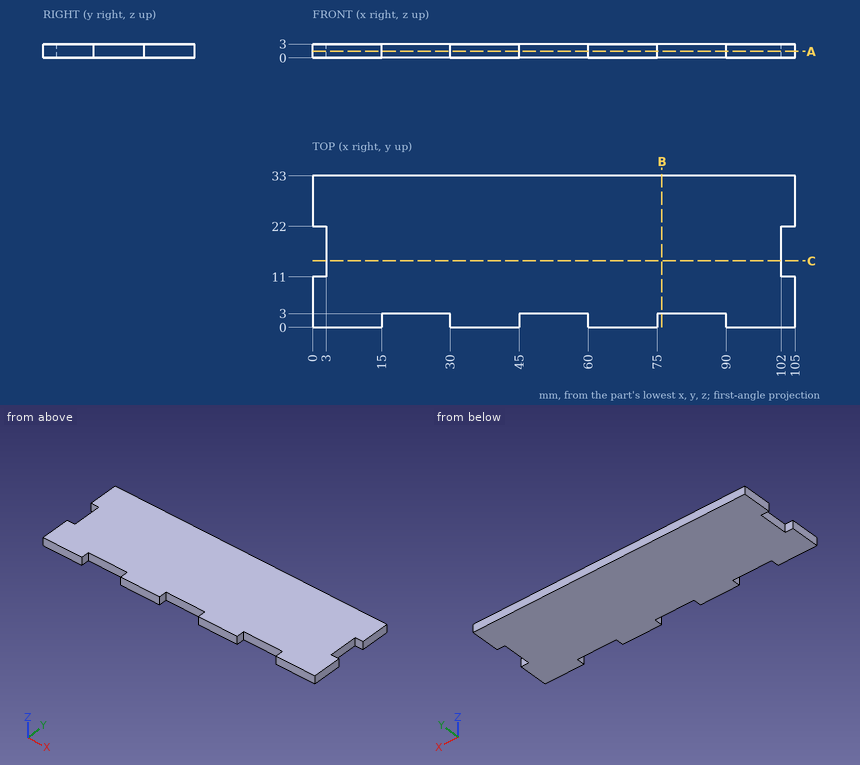
Verification items for this drawing (mm, ordinates from the low corner). Round coordinates to 2 decimals unless told otherwise and drop trailing zeros. Loops run counter-clockwise (first coordinate to the right, second up) from the corner with the lowest first, then second, coordinate; pieces in that order, holes last. Notation, with made-up numbers: (67.25, -5) - (87.25, -5) arc R17 cw to (87.25, 28) - close; hole circle Ø6 at (77, -6.75). An arc over 180 degrees is marked (long way). Answer as CSV lines item,"result". Start each with the question number.
Item 1: Scan lines: line 1 (X direction, y = 14, z = 1.7); line 2 (Y direction, x = 24, z = 2.85). Record each from-to range of solid material in increasing order. Write a range as [from, to].
Item 2: Depth check by flat-ended pin: P1, Ø1.5, axis at x = 83.5, z = 1.5, coming from the -Y side; P2, Ø12, axis at x = 79, y = 17.5, coming from the -Z side. Enter the tip coordinate at first touch or a pass-through.
Item 3: Section check C-C (y = 14.5). Record the boundary of the cut face in (x, z), and give its area (3 significant figures).
Item 4: Section check A-A (z = 1.4). Record the boundary of the cut face in (x, y), and give its area (3 significant figures).
Item 5: Section check B-B (x = 76). Record the boundary of the cut face in (y, z).
Report:
1,line 1,"x = [3, 102]"
1,line 2,"y = [3, 33]"
2,P1,"stops at y = 3"
2,P2,"stops at z = 0"
3,outline,"(3, 0) - (102, 0) - (102, 3) - (3, 3) - close"
3,area,"297 mm2"
4,outline,"(0, 0) - (15, 0) - (15, 3) - (30, 3) - (30, 0) - (45, 0) - (45, 3) - (60, 3) - (60, 0) - (75, 0) - (75, 3) - (90, 3) - (90, 0) - (105, 0) - (105, 11) - (102, 11) - (102, 22) - (105, 22) - (105, 33) - (0, 33) - (0, 22) - (3, 22) - (3, 11) - (0, 11) - close"
4,area,"3,260 mm2"
5,outline,"(3, 0) - (33, 0) - (33, 3) - (3, 3) - close"
